from build123d import *

# Parameters (mm, degrees)
F0_R     = 19.685
F0_R_2   = 10.16
F1_DEPTH = 16.51
F3_T     = -2.54
F2_R     = 10.16
F4_DEPTH = 1.27
F0_R_3   = 1.905
F5_DEPTH = 25.4
F0_R_4   = 3.175
F6_DEPTH = 10.16


with BuildPart() as f1:
    # F0 (on Front) → F1 (new body)
    with BuildSketch(Plane.XZ):
        Circle(F0_R)
        Circle(F0_R_2, mode=Mode.SUBTRACT)
    extrude(amount=F1_DEPTH)

    # F3
    f3_openings = [f1.faces().sort_by_distance(p)[0] for p in [
        (-19.128224, 0, 0),
    ]]
    offset(amount=F3_T, openings=f3_openings)

    # F2 (on face) → F4 (join)
    with BuildSketch(Plane.XZ):
        Circle(F2_R)
    extrude(amount=F4_DEPTH)

    # F0 (on Front) → F5 (cut)
    with BuildSketch(Plane.XZ):
        with Locations((4.490128, 4.490128)):
            Circle(F0_R_3)
        with Locations((6.35, 0)):
            Circle(F0_R_3)
        with Locations((4.490128, -4.490128)):
            Circle(F0_R_3)
        with Locations((0, -6.35)):
            Circle(F0_R_3)
        with Locations((-4.490128, -4.490128)):
            Circle(F0_R_3)
        with Locations((-6.35, 0)):
            Circle(F0_R_3)
        with Locations((-4.490128, 4.490128)):
            Circle(F0_R_3)
        with Locations((0, 6.35)):
            Circle(F0_R_3)
    extrude(amount=F5_DEPTH, mode=Mode.SUBTRACT)

    # F0 (on Front) → F6 (join)
    with BuildSketch(Plane.XZ):
        Circle(F0_R_4)
        Circle(F0_R_3, mode=Mode.SUBTRACT)
    extrude(amount=-F6_DEPTH)


solid = f1.part
Design review of the part built by this model. Coordinates are the model's own, in mm. A direction names the side the tool comes from. Coordinates: 2 decimals unless noted, no trailing zeros. Order: outer loops, then holes, each group sorted by start corner. A loop starts at its lowest first (then second) coordinate and runs counter-clockwise, first axis right, second up. Notation, with made-up numbers: M 74.5,-25.5 L 102.5,-25.5 A21 cw 102.5,-0.5 Z; hole C 83.25,50 d11. An arc over 180 degrees is marked long. Use a Markdown table: item, result.
(1) Add section D-D (z = -5.5). Give the boundary of the cut face in (x, y), then the cut area to 3 significant figures.
Worked answers:
| item | result |
|---|---|
| outline | M -18.9,-16.51 L -8.54,-16.51 L -8.54,-1.27 L -6.11,-1.27 L -6.11,0 L -11.45,0 L -11.45,-13.97 L -16.24,-13.97 L -16.24,0 L -18.9,0 Z; M -2.87,-1.27 L -1.7,-1.27 L -1.7,0 L -2.87,0 Z; M 1.7,-1.27 L 2.87,-1.27 L 2.87,0 L 1.7,0 Z; M 6.11,-1.27 L 8.54,-1.27 L 8.54,-16.51 L 18.9,-16.51 L 18.9,0 L 16.24,0 L 16.24,-13.97 L 11.45,-13.97 L 11.45,0 L 6.11,0 Z |
| area | 217 mm2 |
(2) Add section C-C (y = -2). Give the boundary of the cut face in (x, z) (3 decimals), then the cut area to 3 significant figures.
Worked answers:
| item | result |
|---|---|
| outline | C 0,0 d39.37; C 0,0 d25.4; hole C 0,0 d34.29; hole C 0,0 d20.32 |
| area | 476 mm2 |
(3) Wall thickness on probe 1 along Z at (x, y) = (0, -5) (3 decimals); probe 2 along X at (y, z) = (-3.75, 11); probe 3 along Z at (x, y) = (0, 3) (3 decimals): over which ranges is each line inside the solid? List them lowest first.
Worked answers:
| item | result |
|---|---|
| probe 1 | z = -19.685 to -17.145, -12.7 to -10.16, 10.16 to 12.7, 17.145 to 19.685 |
| probe 2 | x = -16.32 to -13.15, -6.35 to 6.35, 13.15 to 16.32 |
| probe 3 | z = -3.175 to -1.905, 1.905 to 3.175 |
(4) Draft analysis for pull direction Z (two halves, no side actions). For faces 4 (the flat face through (3, 0, -3)), 5 (the cylindrical face through (-15.62, -8.14, -11.98)), 6 (the cylindrical face through (2.98, -0.63, -5.65)), state which applies: released by +Z, released by -Z, zero draft, split by the parting line, or undercut.
Worked answers:
| item | result |
|---|---|
| face 4 | zero draft |
| face 5 | split by the parting line |
| face 6 | undercut |
(5) For P1, Ø3.5, axis at x = -4.49, z = 4.49, coming from the +Y side; P2, Ø2, axis at x = -1, y = 6, coming from the +Z side (3 decimals); P3, Ø3, axis at y = -5.5, z = -3.5, coming from the -X side; P4, Ø1.9, axis at x = -0.5, z = 0.5, coming from the +Y side, all flat-tipped, find the tip position at first contact; note any pin that passes through.
Worked answers:
| item | result |
|---|---|
| P1 | passes through |
| P2 | stops at z = 3.175 |
| P3 | stops at x = -19.58 |
| P4 | stops at y = 0 |
(6) For faces 1 (the cylindrical face through (-3.61, -0.63, -6.18)), 2 (the flat face through (0, -1.27, 0)), 3 (the flat face through (0, 0, 0)), list the 3-axis set-ups (+Z, -Z, +X, -X, +Y, -Y) from which the entire face can be reached by the end or side of a thin tool; tool diameter is ignored.
Worked answers:
| item | result |
|---|---|
| face 1 | +Y, -Y |
| face 2 | -Y |
| face 3 | +Y |
(7) Add section A-A (x = 0). Count the separate pieces of the cut face and the enclosed holes in it, then the cut area to 3 significant figures.
Worked answers:
| item | result |
|---|---|
| separate pieces | 3 |
| enclosed holes | 0 |
| area | 232 mm2 |
